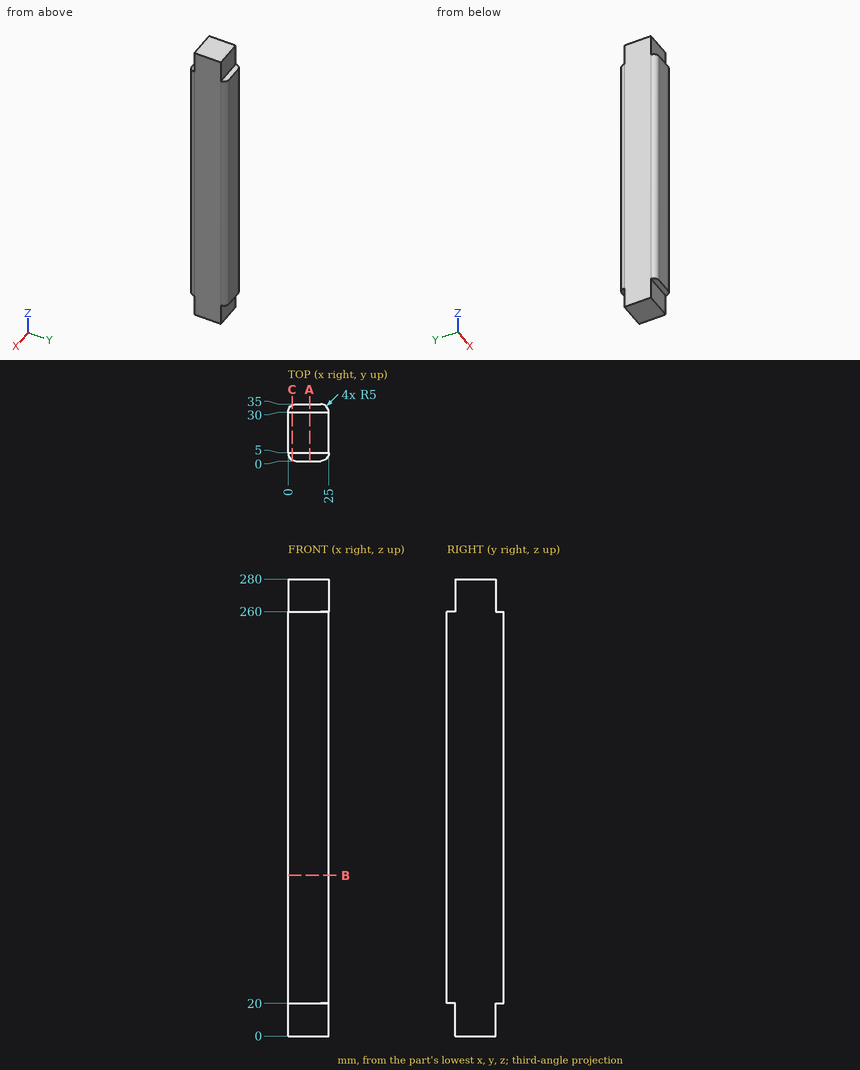
Design review of the part shown in the three views and the two pictorial views. Dimensions are in mm from the part's minimum x, y and z. Coordinates: 2 decimals unless noted, no trailing zeros. Order: outer loops, then holes, each group sorted by start corner. A loop starts at its lowest first (then second) coordinate and runs counter-clockwise, first axis right, second up. Notation, with made-up numbers: (27.25, 81.5) -> (46.25, 81.5) arc R16 cw to (46.25, 94.5) -> close; hole circle Ø8 at (-25, -3). An arc over 180 degrees is marked (long way). Use one line per item in the form item = value. Start each with the question number.
(1) Add section C-C on x = 2.5. State the section outline as (y, z) points.
(2) Insertion check: pin 1 (1.5 mm diameter, centred on x = 3, y = 30.5, fed in from +Z); pin 2 (1.5 mm diameter, centred on x = 8.5, y = 3.5, fed in from +Z); pin 3 (6 mm diameter, centred on x = 11.5, z = 273, fed in from -Y). Each pin has a flat end and moves straight along its axis. Give the tip position at first contact, or say it passes through.
(3) Add section A-A on x = 13.25. State the section outline as (y, z) points, plus the area to 3 significant figures.
(4) For probe 1 along Y at (x, z) = (4.75, 187); probe 2 along X at (y, z) = (32, 201); probe 3 along X at (y, z) = (33, 205), list the stretches that pass through material, from the lowest coordinate up.
(5) Add section B-B on z = 98.5. State the section outline as (x, y) points, plus the area to 3 significant figures.
Answer block:
q1.outline = (0.67, 20) -> (5, 20) -> (5, 0) -> (30, 0) -> (30, 20) -> (34.33, 20) -> (34.33, 260) -> (30, 260) -> (30, 280) -> (5, 280) -> (5, 260) -> (0.67, 260) -> close
q2.pin_1 = 280
q2.pin_2 = 260
q2.pin_3 = 5
q3.outline = (0, 20) -> (5, 20) -> (5, 0) -> (30, 0) -> (30, 20) -> (35, 20) -> (35, 260) -> (30, 260) -> (30, 280) -> (5, 280) -> (5, 260) -> (0, 260) -> close
q3.area = 9,400 mm²
q4.probe_1 = 0.01 to 34.99
q4.probe_2 = 0.42 to 24.58
q4.probe_3 = 1 to 24
q5.outline = (0, 5) arc R5 ccw to (5, 0) -> (20, 0) arc R5 ccw to (25, 5) -> (25, 30) arc R5 ccw to (20, 35) -> (5, 35) arc R5 ccw to (0, 30) -> close
q5.area = 854 mm²
